```python
from build123d import *

# Parameters (mm, degrees)
F1_DEPTH = 3.175


# Not quite as in the source:
# - a length typed as a fraction of an inch, garbled in the dataset ("3 / 203.2 mm" for 3/8 in), is restored


with BuildPart() as f1:
    # F0 (on Top) → F1 (new body)
    with BuildSketch(Plane.XY):
        with BuildLine():
            ThreePointArc((-4.7624995714, 0.0020204955), (-4.528844398, 1.4734227733), (-3.8519931198, 2.800634795))
            Line((-3.8519931198, 2.800634795), (-40.7900391434, 29.6568553891))
            ThreePointArc((-40.7900391434, 29.6568553891), (-52.8581727457, 19.1196962374), (-68.3027796686, 14.8610945149))
            ThreePointArc((-68.3027796686, 14.8610945149), (-69.202037382, 9.8589990779), (-69.7354707037, 4.8047857774))
            Line((-69.7354707037, 4.8047857774), (-35.4708737874, 4.7902489857))
            ThreePointArc((-35.4708737874, 4.7902489857), (-31.7421994573, 3.5901618172), (-30.1466961845, 0.012789768))
            Line((-30.1466961845, 0.012789768), (-4.7624995714, 0.0020204955))
        make_face()
        with BuildLine():
            ThreePointArc((-3.8519931198, 2.800634795), (-2.7981829099, 3.853774598), (-1.4705404248, 4.5297811326))
            Line((-1.4705404248, 4.5297811326), (-9.3085437064, 28.6735848558))
            ThreePointArc((-9.3085437064, 28.6735848558), (-13.2035838045, 29.0881739368), (-15.4950023114, 32.2650627762))
            Line((-15.4950023114, 32.2650627762), (-26.0750504874, 64.8553280982))
            ThreePointArc((-26.0750504874, 64.8553280982), (-30.7184565015, 62.789316534), (-35.1994748016, 60.3913802983))
            ThreePointArc((-35.1994748016, 60.3913802983), (-34.4878638746, 44.3862192082), (-40.7900391434, 29.6568553891))
            Line((-40.7900391434, 29.6568553891), (-3.8519931198, 2.800634795))
        make_face()
        with BuildLine():
            ThreePointArc((-1.4705404248, 4.5297811326), (0.0010102478, 4.7624998929), (1.4724620567, 4.5291568466))
            Line((1.4724620567, 4.5291568466), (15.5923915392, 47.9607515681))
            ThreePointArc((15.5923915392, 47.9607515681), (1.8403043285, 56.1797338033), (-6.9847818286, 69.5509501261))
            ThreePointArc((-6.9847818286, 69.5509501261), (-12.0198259563, 68.8596080777), (-16.9913293895, 67.8042518299))
            Line((-16.9913293895, 67.8042518299), (-6.4112812135, 35.213986508))
            ThreePointArc((-6.4112812135, 35.213986508), (-6.3997434798, 31.296961061), (-9.3085437064, 28.6735848558))
            Line((-9.3085437064, 28.6735848558), (-1.4705404248, 4.5297811326))
        make_face()
        with BuildLine():
            ThreePointArc((1.4724620567, 4.5291568466), (2.7998176259, 3.8525871193), (3.8531809453, 2.7990003309))
            Line((3.8531809453, 2.7990003309), (24.390695172, 17.7177155255))
            ThreePointArc((24.390695172, 17.7177155255), (23.5807088667, 21.5500964639), (25.893485986, 24.7114701318))
            Line((25.893485986, 24.7114701318), (53.6158384941, 44.8493445127))
            ThreePointArc((53.6158384941, 44.8493445127), (50.2154123333, 48.626476377), (46.5495312326, 52.1465529318))
            ThreePointArc((46.5495312326, 52.1465529318), (31.5485727352, 46.5213581982), (15.5923915392, 47.9607515681))
            Line((15.5923915392, 47.9607515681), (1.4724620567, 4.5291568466))
        make_face()
        with BuildLine():
            Line((24.390695172, 17.7177155255), (3.8531809453, 2.7990003309))
            ThreePointArc((3.8531809453, 2.7990003309), (4.5294690915, 1.4715012738), (4.7625, 0))
            Line((4.7625, 0), (50.4317, 0))
            ThreePointArc((50.4317, 0), (53.9961373847, 15.6194224529), (63.9836925433, 28.1462063014))
            ThreePointArc((63.9836925433, 28.1462063014), (61.7694966371, 32.7208057029), (59.2287671577, 37.1224323236))
            Line((59.2287671577, 37.1224323236), (31.5064146496, 16.9845579428))
            ThreePointArc((31.5064146496, 16.9845579428), (27.7848747553, 15.7625259109), (24.390695172, 17.7177155255))
        make_face()
        with BuildLine():
            Line((50.4317, 0), (4.7625, 0))
            ThreePointArc((4.7625, 0), (3.8519931198, -2.800634795), (1.4686185281, -4.5304046032))
            Line((1.4686185281, -4.5304046032), (15.5516911338, -47.9739644784))
            ThreePointArc((15.5516911338, -47.9739644784), (31.509087914, -46.5481104778), (46.5052680226, -52.1860315294))
            ThreePointArc((46.5052680226, -52.1860315294), (50.1741345955, -48.6690667492), (53.5777644361, -44.8948215128))
            Line((53.5777644361, -44.8948215128), (25.8725089337, -24.7334319103))
            ThreePointArc((25.8725089337, -24.7334319103), (24.3756528753, -17.7384047006), (31.491991877, -17.0112850838))
            Line((31.491991877, -17.0112850838), (59.1972473794, -37.1726746864))
            ThreePointArc((59.1972473794, -37.1726746864), (61.7556092427, -32.7470085305), (63.9836925433, -28.1462063014))
            ThreePointArc((63.9836925433, -28.1462063014), (53.9961373847, -15.6194224529), (50.4317, 0))
        make_face()
        with BuildLine():
            ThreePointArc((1.4686185281, -4.5304046032), (-0.0030307432, -4.7624990357), (-1.4743834236, -4.5285317455))
            Line((-1.4743834236, -4.5285317455), (-9.3328699489, -28.6656762162))
            ThreePointArc((-9.3328699489, -28.6656762162), (-6.4262967093, -31.2915195998), (-6.4411580428, -35.208533847))
            Line((-6.4411580428, -35.208533847), (-17.0488553147, -67.7898102453))
            ThreePointArc((-17.0488553147, -67.7898102453), (-12.078249143, -68.8493844437), (-7.0437934329, -69.5449984881))
            ThreePointArc((-7.0437934329, -69.5449984881), (1.7926350508, -56.1812750817), (15.5516911338, -47.9739644784))
            Line((15.5516911338, -47.9739644784), (1.4686185281, -4.5304046032))
        make_face()
        with BuildLine():
            ThreePointArc((-1.4743834236, -4.5285317455), (-2.801451838, -3.851398947), (-3.8543680773, -2.797365363))
            Line((-3.8543680773, -2.797365363), (-40.8151883603, -29.6222342844))
            ThreePointArc((-40.8151883603, -29.6222342844), (-34.5255132545, -44.3569402094), (-35.2507043361, -60.3614917348))
            ThreePointArc((-35.2507043361, -60.3614917348), (-30.7717223028, -62.7632292601), (-26.130070975, -64.8331800198))
            Line((-26.130070975, -64.8331800198), (-15.5223737031, -32.2519036214))
            ThreePointArc((-15.5223737031, -32.2519036214), (-13.2282604246, -29.0769601987), (-9.3328699489, -28.6656762162))
            Line((-9.3328699489, -28.6656762162), (-1.4743834236, -4.5285317455))
        make_face()
        with BuildLine():
            ThreePointArc((-3.8543680773, -2.797365363), (-4.5300929698, -1.4695795095), (-4.7624995714, 0.0020204955))
            Line((-4.7624995714, 0.0020204955), (-30.1466961845, 0.012789768))
            ThreePointArc((-30.1466961845, 0.012789768), (-31.7452342902, -3.5632272058), (-35.4749255544, -4.7601501548))
            Line((-35.4749255544, -4.7601501548), (-69.7395224707, -4.7456133631))
            ThreePointArc((-69.7395224707, -4.7456133631), (-69.210377851, -9.8002774634), (-68.3153647492, -14.8031341217))
            ThreePointArc((-68.3153647492, -14.8031341217), (-52.874376818, -19.0748390906), (-40.8151883603, -29.6222342844))
            Line((-40.8151883603, -29.6222342844), (-3.8543680773, -2.797365363))
        make_face()
    extrude(amount=F1_DEPTH)


solid = f1.part
```
Model file for the job. Use its own axes, mm. A direction names the side the tool comes from. Give positions to 0.01 mm unless a question says otherwise; leave off trailing zeros. Order: outer loops, then holes, each group sorted by start corner. A loop starts at its lowest first (then second) coordinate and runs counter-clockwise, first axis right, second up.
1) Wall check: probe 1 along X at (y, z) = (33.5, 2.8) (3 decimals); probe 2 along Y at (x, z) = (37.5, 1.7); probe 3 along X at (y, z) = (-32.5, 1.3). Give the ranges that are in metal, low to high.
2) Saw through at C-C, the plane y = 26.5. Write the cut outline in (x, z) (3 decimals), then the cut area to 3 significant figures.
3) Mould opens along X. For faces 3 (the flat face through (39.56, 34.64, 1.57)), 4 (the flat face through (39.919, -34.955, 1.565)), 5 (the cylindrical face through (50.26, 48.58, 1.57)), 6 (the cylindrical face through (-69.22, -9.73, 1.57)) say: +X half, -X half, draft (parallel to the pull), parting line (faces both ways), or undercut.
4) Pin check, flat tips, straight feed: pin 1 (1.5 mm diameter, centred on y = -24, z = 3, fed in from -X); pin 2 (1 mm diameter, centred on x = -51, z = 2.5, fed in from -Y). Stop position of each tip, or through.
5) Saw through at B-B, the plane x = 38.5. Write the cut outline in (y, z) (3 decimals), then the cut area to 3 significant figures.
6) Saw through at D-D, the plane x = 7. Write the cut outline in (y, z) (3 decimals), then the cut area to 3 significant figures.
7) 3-axis set-ups, long thin cutter, end or side, ignore diameter. For faces 1 (the flat face through (-11.775, 51.737, 1.565)), 2 (the flat face through (11, 1, 3.175)): which of +Z, -Z, +X, -X, +Y, -Y reach the whole face in a straight line?
8) Saw through at A-A, the plane y = 57. Write the cut outline in (x, z) (3 decimals).
Computed:
1. probe 1: x = -38.352 to -15.896, -5.995 to 37.992, 54.242 to 61.35
1. probe 2: y = -47.89 to -33.19, -21.38 to 21.34, 33.14 to 47.85
1. probe 3: x = -38.93 to -15.6, -6.07 to 36.55, 52.78 to 61.89
2. outline: (-43.371, 0) - (28.356, 0) - (28.356, 3.175) - (-43.371, 3.175) - close; (44.606, 0) - (62.063, 0) - (62.063, 3.175) - (44.606, 3.175) - close
2. area: 283 mm2
3. face 3: undercut
3. face 4: undercut
3. face 5: +X half
3. face 6: -X half
4. pin 1: stops at x = -46.74
4. pin 2: stops at y = -20.47
5. outline: (-48.224, 0) - (-33.923, 0) - (-33.923, 3.175) - (-48.224, 3.175) - close; (-22.111, 0) - (22.065, 0) - (22.065, 3.175) - (-22.111, 3.175) - close; (33.869, 0) - (48.177, 0) - (48.177, 3.175) - (33.869, 3.175) - close
5. area: 231 mm2
6. outline: (-52.057, 0) - (52.08, 0) - (52.08, 3.175) - (-52.057, 3.175) - close
6. area: 331 mm2
7. face 1: +Z, -Z
7. face 2: +Z, +X, -X, +Y, -Y
8. outline: (-34.439, 0) - (-23.525, 0) - (-23.525, 3.175) - (-34.439, 3.175) - close; (-13.484, 0) - (1.01, 0) - (1.01, 3.175) - (-13.484, 3.175) - close
